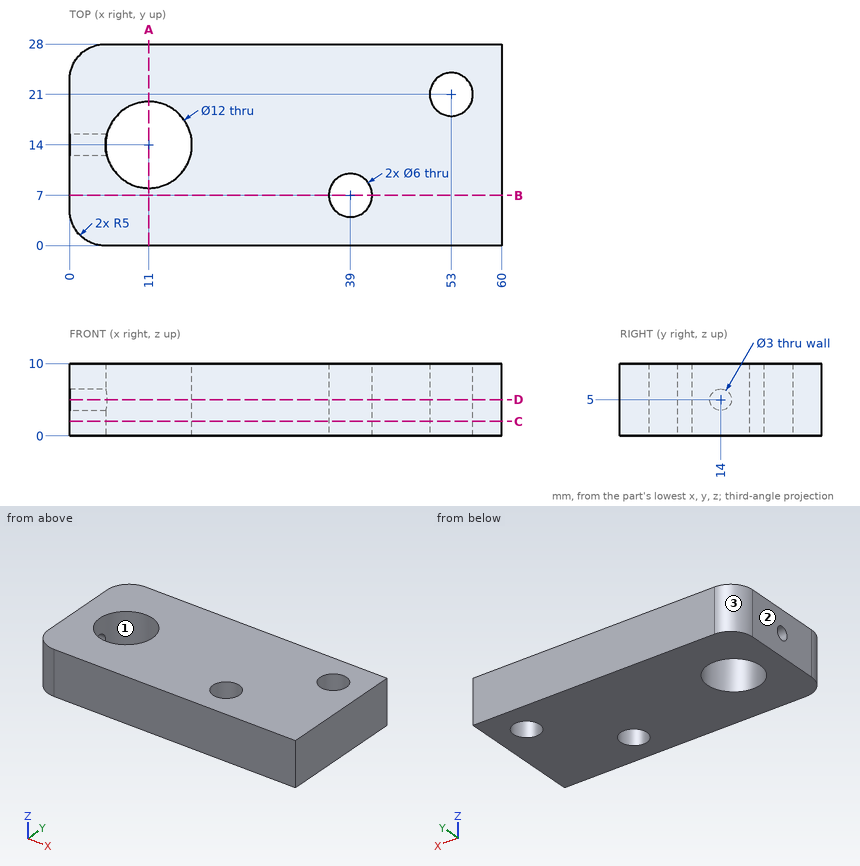
Design review of the part shown in the three views and the two pictorial views. Dimensions are in mm from the part's minimum x, y and z. Give positions to 0.01 mm unless a question says otherwise; leave off trailing zeros. Loops run counter-clockwise (first coordinate to the right, second up) from the corner with the lowest first, then second, coordinate; pieces in that order, holes last. Notation, with made-up numbers: M 34.25,85.25 L 43.25,85.25 A15 ccw 43.25,106.25 Z; hole C 2,-12.75 d5. An arc over 180 degrees is marked long. Write item = value, one per line.
Q1. To check wall thickness, follow line 1 (Z direction, x = 3.25, y = 14); line 2 (Y direction, x = 53, z = 2.25); line 3 (Y direction, x = 11, z = 3). State the ranges of each line that lie inside material, in increasing order. Write a range as [from, to].
Output values:
line_1 = [0, 3.5], [6.5, 10]
line_2 = [0, 18], [24, 28]
line_3 = [0, 8], [20, 28]
Q2. Draft analysis for pull direction Y (two halves, no side actions). For the marked faces 1, 2 and 3, state which applies: +Y half, -Y half, draft (parallel to the pull), parting line (faces both ways), or undercut.
Output values:
face_1 = undercut
face_2 = draft
face_3 = +Y half
Q3. We need section C-C (z = 2). Give the boundary of the cut face in (x, y), plus the area to 3 significant figures.
Output values:
outline = M 0,5 A5 ccw 5,0 L 60,0 L 60,28 L 5,28 A5 ccw 0,23 Z; hole C 11,14 d12; hole C 39,7 d6; hole C 53,21 d6
area = 1,500 mm^2
Q4. We need section A-A (x = 11). Give the boundary of the cut face in (y, z), plus the area to 3 significant figures.
Output values:
outline = M 0,0 L 8,0 L 8,10 L 0,10 Z; M 20,0 L 28,0 L 28,10 L 20,10 Z
area = 160 mm^2
Q5. We need section B-B (y = 7). Give the boundary of the cut face in (x, z).
Output values:
outline = M 0,0 L 36,0 L 36,10 L 0,10 Z; M 42,0 L 60,0 L 60,10 L 42,10 Z
Q6. We need section D-D (z = 5). Give the boundary of the cut face in (x, y).
Output values:
outline = M 0,5 A5 ccw 5,0 L 60,0 L 60,28 L 5,28 A5 ccw 0,23 L 0,15.5 L 5.19,15.5 A6 cw long 5.19,12.5 L 0,12.5 Z; hole C 39,7 d6; hole C 53,21 d6
Q7. Insertion check: pin 1 (6 mm diameter, centred on x = 52, z = 7.5, fed in from -Y); pin 2 (1.5 mm diameter, centred on y = 24.5, z = 6.5, fed in from -X); pin 3 (2.5 mm diameter, centred on y = 14, z = 5, fed in from -X). Each pin has a flat end and moves straight along its axis. Give the tip position at first contact, or say it passes through.
Output values:
pin_1 = 0
pin_2 = 0.06
pin_3 = 16.87
